```python
from build123d import *

# Parameters (mm, degrees)
F0_R     = 1.60312
F0_W     = 6.4
F0_H     = 3.4
F1_DEPTH = 3


# Not quite as in the source:
# - ends of sketch curves that miss each other by under 0.0002 mm in the source are joined


with BuildPart() as f1:
    # F0 (on Top) → F1 (new body)
    with BuildSketch(Plane.XY):
        with BuildLine():
            ThreePointArc((17.5, -2.6), (14.9, 0), (17.5, 2.6))
            Line((17.5, 2.6), (30.5, 2.6))
            ThreePointArc((30.5, 2.6), (31.2071067812, 2.8928932188), (31.5, 3.6))
            Line((31.5, 3.6), (31.5, 12.5))
            Line((31.5, 12.5), (24.2543, 30.6142))
            ThreePointArc((24.2543, 30.6142), (23.1507874279, 31.9842016914), (21.468901, 32.5))
            Line((21.468901, 32.5), (-28.5, 32.5))
            ThreePointArc((-28.5, 32.5), (-30.6213203436, 31.6213203436), (-31.5, 29.5))
            Line((-31.5, 29.5), (-31.5, -29.5))
            ThreePointArc((-31.5, -29.5), (-30.6213203436, -31.6213203436), (-28.5, -32.5))
            Line((-28.5, -32.5), (21.468901, -32.5))
            ThreePointArc((21.468901, -32.5), (23.1507874279, -31.9842016914), (24.2543310727, -30.6141720291))
            Line((24.2543310727, -30.6141720291), (31.5, -12.5))
            Line((31.5, -12.5), (31.5, -3.6))
            ThreePointArc((31.5, -3.6), (31.2071067812, -2.8928932188), (30.5, -2.6))
            Line((30.5, -2.6), (17.5, -2.6))
        make_face()
        with Locations((-28.5, -28.5)):
            Circle(F0_R, mode=Mode.SUBTRACT)
        with Locations((-21.5, -28)):
            Rectangle(F0_W, F0_H, mode=Mode.SUBTRACT)
        with Locations((-21.5, -17)):
            Rectangle(F0_W, F0_H, mode=Mode.SUBTRACT)
        with Locations((-14.5, -16.8)):
            Circle(F0_R, mode=Mode.SUBTRACT)
        with BuildLine():
            ThreePointArc((0.5, -23.5), (-0.0857864376, -24.9142135624), (-1.5, -25.5))
            Line((-1.5, -25.5), (-6.5, -25.5))
            ThreePointArc((-6.5, -25.5), (-7.9142135624, -24.9142135624), (-8.5, -23.5))
            Line((-8.5, -23.5), (-8.5, -7))
            ThreePointArc((-8.5, -7), (-7.9142135624, -5.5857864376), (-6.5, -5))
            Line((-6.5, -5), (-1.5, -5))
            ThreePointArc((-1.5, -5), (-0.0857864376, -5.5857864376), (0.5, -7))
            Line((0.5, -7), (0.5, -23.5))
        make_face(mode=Mode.SUBTRACT)
        with Locations((13.5, -28)):
            Rectangle(F0_W, F0_H, mode=Mode.SUBTRACT)
        with Locations((6.5, -16.8)):
            Circle(F0_R, mode=Mode.SUBTRACT)
        with Locations((13.5, -17)):
            Rectangle(F0_W, F0_H, mode=Mode.SUBTRACT)
        with Locations((20.5, -28.5)):
            Circle(F0_R, mode=Mode.SUBTRACT)
        with BuildLine():
            ThreePointArc((-1.5, 25.5), (-0.0857864376, 24.9142135624), (0.5, 23.5))
            Line((0.5, 23.5), (0.5, 7))
            ThreePointArc((0.5, 7), (-0.0857864376, 5.5857864376), (-1.5, 5))
            Line((-1.5, 5), (-6.5, 5))
            ThreePointArc((-6.5, 5), (-7.9142135624, 5.5857864376), (-8.5, 7))
            Line((-8.5, 7), (-8.5, 23.5))
            ThreePointArc((-8.5, 23.5), (-7.9142135624, 24.9142135624), (-6.5, 25.5))
            Line((-6.5, 25.5), (-1.5, 25.5))
        make_face(mode=Mode.SUBTRACT)
        with Locations((-21.5, 17)):
            Rectangle(F0_W, F0_H, mode=Mode.SUBTRACT)
        with Locations((-28.5, 28.5)):
            Circle(F0_R, mode=Mode.SUBTRACT)
        with Locations((-21.5, 28)):
            Rectangle(F0_W, F0_H, mode=Mode.SUBTRACT)
        with Locations((-14.5, 16.8)):
            Circle(F0_R, mode=Mode.SUBTRACT)
        with Locations((6.5, 16.8)):
            Circle(F0_R, mode=Mode.SUBTRACT)
        with Locations((13.5, 17)):
            Rectangle(F0_W, F0_H, mode=Mode.SUBTRACT)
        with Locations((13.5, 28)):
            Rectangle(F0_W, F0_H, mode=Mode.SUBTRACT)
        with Locations((20.5, 28.5)):
            Circle(F0_R, mode=Mode.SUBTRACT)
    extrude(amount=F1_DEPTH)


solid = f1.part
```
Geometry: final body of the model. Coordinates: model frame, mm. A direction names the side the tool comes from. Coordinates: 2 decimals unless noted, no trailing zeros. Order: outer loops, then holes, each group sorted by start corner. A loop starts at its lowest first (then second) coordinate and runs counter-clockwise, first axis right, second up.
Item 1: Section query B-B (y = -28.5). Output: boundary loops of the cut face in (x, z).
Answer:
outline: (-31.5, 0) - (-30.1, 0) - (-30.1, 3) - (-31.5, 3) - close; (-26.9, 0) - (-24.7, 0) - (-24.7, 3) - (-26.9, 3) - close; (-18.3, 0) - (10.3, 0) - (10.3, 3) - (-18.3, 3) - close; (16.7, 0) - (18.9, 0) - (18.9, 3) - (16.7, 3) - close; (22.1, 0) - (25.1, 0) - (25.1, 3) - (22.1, 3) - close
Item 2: Section query A-A (x = 20.5). Output: boundary loops of the cut face in (y, z).
Answer:
outline: (-32.5, 0) - (-30.1, 0) - (-30.1, 3) - (-32.5, 3) - close; (-26.9, 0) - (-2.6, 0) - (-2.6, 3) - (-26.9, 3) - close; (2.6, 0) - (26.9, 0) - (26.9, 3) - (2.6, 3) - close; (30.1, 0) - (32.5, 0) - (32.5, 3) - (30.1, 3) - close
Item 3: Material intervals for line 1 along Y through (x, z) = (-28.5, 2.3); line 2 along X through (y, z) = (-17, 0.55); line 3 along Y through (x, z) = (20.5, 0.75), sorted ascending.
Answer:
line 1: y = -32.5 to -30.1, -26.9 to 26.9, 30.1 to 32.5
line 2: x = -31.5 to -24.7, -18.3 to -16.09, -12.91 to -8.5, 0.5 to 4.91, 8.09 to 10.3, 16.7 to 29.7
line 3: y = -32.5 to -30.1, -26.9 to -2.6, 2.6 to 26.9, 30.1 to 32.5
Item 4: Section query D-D (x = -14.5). Output: boundary loops of the cut face in (y, z), then the cut area to 3 significant figures.
Answer:
outline: (-32.5, 0) - (-18.4, 0) - (-18.4, 3) - (-32.5, 3) - close; (-15.2, 0) - (15.2, 0) - (15.2, 3) - (-15.2, 3) - close; (18.4, 0) - (32.5, 0) - (32.5, 3) - (18.4, 3) - close
area: 176 mm2
Item 5: Draft query along Y for faces 1 (the face through (27.83, -21.68, 1.48)), 2 (the face through (-30.6, 31.64, 1.48)), 3 (the face through (-7.93, 24.9, 1.48)), 4 (the face through (-0.1, 24.93, 1.48)). Return one class per face: released by +Y, released by -Y, zero draft, split by the parting line, or undercut.
Answer:
face 1: released by -Y
face 2: released by +Y
face 3: undercut
face 4: undercut
Item 6: Contact query for flat-ended pins moving along their axis: P1, Ø8, axis at x = 20.5, y = -21, coming from the -Z side; P2, Ø0.9, axis at y = 16, z = 2, coming from the +X side; P3, Ø1.5, axis at y = -16.5, z = 1, coming from the +X side; P4, Ø1.9, axis at x = -14.5, y = -16.8, coming from the +Z side. Output: stop coordinate, or through.
Answer:
P1: stops at z = 0
P2: stops at x = 30.28
P3: stops at x = 30.2
P4: passes through
Item 7: Access query for faces 5 (the face through (16.7, -28, 1)), 6 (the face through (-31.5, 0, 1)). Directions: +Z, -Z, +X, -X, +Y, -Y. A direction counts if a zero-diameter tool reaches every point of the face in a straight line with its end or side. Return the directions, or none.
Answer:
face 5: +Z, -Z
face 6: +Z, -Z, -X, +Y, -Y
Item 8: Section query C-C (y = 16.8). Output: boundary loops of the cut face in (x, z).
Answer:
outline: (-31.5, 0) - (-24.7, 0) - (-24.7, 3) - (-31.5, 3) - close; (-18.3, 0) - (-16.1, 0) - (-16.1, 3) - (-18.3, 3) - close; (-12.9, 0) - (-8.5, 0) - (-8.5, 3) - (-12.9, 3) - close; (0.5, 0) - (4.9, 0) - (4.9, 3) - (0.5, 3) - close; (8.1, 0) - (10.3, 0) - (10.3, 3) - (8.1, 3) - close; (16.7, 0) - (29.78, 0) - (29.78, 3) - (16.7, 3) - close
